For this review, use the dimensioned drawing (mm, ordinates from the lowest corner) and the shaded views. Give positions to 0.01 mm unless a question says otherwise; leave off trailing zeros. Loops run counter-clockwise (first coordinate to the right, second up) from the corner with the lowest first, then second, coordinate; pieces in that order, holes last. Notation, with made-up numbers: (-11, 77) - (22, 77) arc R20 cw to (22, 116) - close; hole circle Ø7 at (-1.75, -3). An arc over 180 degrees is marked (long way). Write each question's results on one line, items separated by ' | '.
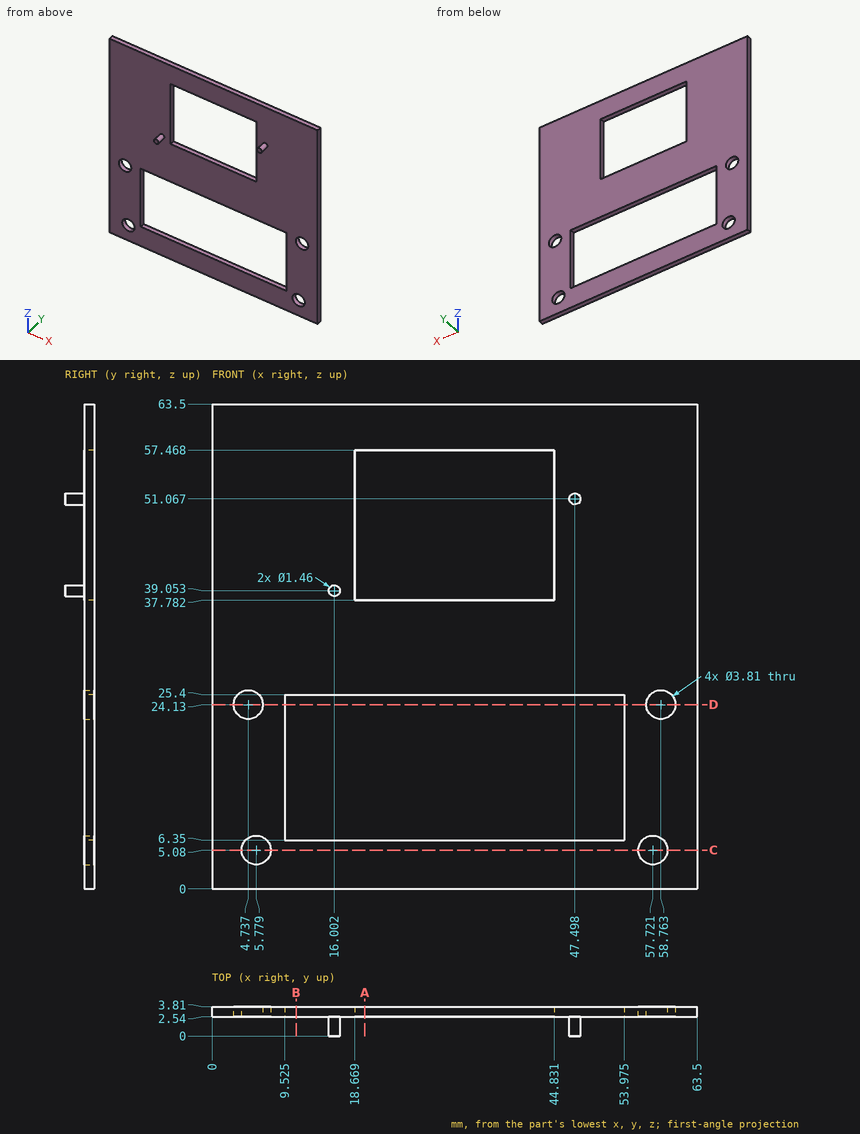
Item 1: We need section B-B on x = 11. Give the boundary of the cut face in (y, z).
Output values:
outline: (2.54, 0) - (3.81, 0) - (3.81, 6.35) - (2.54, 6.35) - close; (2.54, 25.4) - (3.81, 25.4) - (3.81, 63.5) - (2.54, 63.5) - close
Item 2: We need section C-C on z = 5.08. Give the boundary of the cut face in (x, y).
Output values:
outline: (0, 2.54) - (3.87, 2.54) - (3.87, 3.81) - (0, 3.81) - close; (7.68, 2.54) - (55.82, 2.54) - (55.82, 3.81) - (7.68, 3.81) - close; (59.63, 2.54) - (63.5, 2.54) - (63.5, 3.81) - (59.63, 3.81) - close
Item 3: We need section D-D on z = 24.13. Give the boundary of the cut face in (x, y) (1 decimal).
Output values:
outline: (0, 2.5) - (2.8, 2.5) - (2.8, 3.8) - (0, 3.8) - close; (6.6, 2.5) - (9.5, 2.5) - (9.5, 3.8) - (6.6, 3.8) - close; (54, 2.5) - (56.9, 2.5) - (56.9, 3.8) - (54, 3.8) - close; (60.7, 2.5) - (63.5, 2.5) - (63.5, 3.8) - (60.7, 3.8) - close
Item 4: Clearance check with a flat-ended pin moving along its axis: P1, Ø12, axis at x = 39.5, z = 26.5, coming from the -Y side. State where the tip first meets the part, or that it passes through.
Output values:
P1: stops at y = 2.54
Item 5: We need section A-A on x = 20. Give the boundary of the cut face in (y, z).
Output values:
outline: (2.54, 0) - (3.81, 0) - (3.81, 6.35) - (2.54, 6.35) - close; (2.54, 25.4) - (3.81, 25.4) - (3.81, 37.78) - (2.54, 37.78) - close; (2.54, 57.47) - (3.81, 57.47) - (3.81, 63.5) - (2.54, 63.5) - close
Item 6: Wall thickness on probe 1 along X at (y, z) = (3.05, 5.08); probe 2 along Z at (x, y) = (23, 3.35); probe 3 along X at (y, z) = (3.5, 24.13) (1 decimal): over which ranges is each line inside the solid? List them lowest first.
Output values:
probe 1: x = 0 to 3.87, 7.68 to 55.82, 59.63 to 63.5 | probe 2: z = 0 to 6.35, 25.4 to 37.78, 57.47 to 63.5 | probe 3: x = 0 to 2.8, 6.6 to 9.5, 54 to 56.9, 60.7 to 63.5
